Could you check a few things on this model? Use its own coordinates, in mm. A direction names the side the tool comes from. Round coordinates to 2 decimals unless told otherwise and drop trailing zeros. Write each loop counter-clockwise with the first axis right and the second up, starting at its lowest first coordinate (ties: lowest second). Pieces come first, ordered by that corner, then holes. Notation, with made-up numbers: (4.25, -23) - (31.25, -23) arc R28 cw to (31.25, 1) - close; hole circle Ø5 at (-26.75, 16). An arc over 180 degrees is marked (long way). Write each question's results on one line, items separated by ' | '. Start each with the question number.
(1) For P1, Ø2.5, axis at y = 497.5, z = 23.5, coming from the -X side; P2, Ø0.9, axis at y = 539, z = 24.5, coming from the +X side; P3, Ø4, axis at y = 151, z = 21.5, coming from the +X side, each with a flat end and sliding along its axis, tell me the tip position at first contact or that it passes through.
(2) Please list where these lines run through material, in increasing order: line 1 (Z direction, x = 380.5, y = 255); line 2 (X direction, y = 876.5, z = 19); line 3 (X direction, y = 757.5, z = 5.5). Write a range as [from, to].
(3) Imagine slicing it at B-B on y = 354.5. Write out the boundary of the cut face in (x, z), then the cut area to 3 significant figures.
(4) Imagine slicing it at A-A on x = 613. Write out the boundary of the cut face in (y, z).
(5) On a 3-axis mill with a long thin cutter (end or side, diameter ignored), from which of +Z, -Z, +X, -X, +Y, -Y can I reach the whole of each face in a straight line? I mean faces 1 (the flat face through (1002, 618, 25.4)), 2 (the flat face through (664, 618, 3.048)). Say none if no direction works.
(6) Thinking about a two-plate mould opening in Z: for faces 3 (the flat face through (664, 618, 0)), 4 (the flat face through (344, 601, 25.4)), 5 (the flat face through (1011, 618, 22.352)), which applies, +Z half, -Z half, draft (parallel to the pull), parting line (faces both ways), or undercut?
Autodesk Inventor part; units mm, degrees
ref_plane "YZ Plane" through (0, 0, 0) normal (1, 0, 0) x (0, 1, 0)
ref_plane "XZ Plane" through (0, 0, 0) normal (0, 1, 0) x (-1, 0, 0)
ref_plane "XY Plane" through (0, 0, 0) normal (0, 0, 1) x (1, 0, 0)
sketch "Sketch1" plane through (0, 0, 0) normal (0, 0, 1) x (1, 0, 0)
  line L0 (0, 0) -> (1346.2, 0)
  line L1 (1346.2, 0) -> (1346.2, 1219.2)
  line L2 (1346.2, 1219.2) -> (0, 1219.2)
  line L3 (0, 1219.2) -> (0, 0)
  dimension "d0" = 1346.2
  dimension "d1" = 1219.2
extrude "Plate1" add sketch "Sketch1" along normal blind 3.048
sketch "Sketch2" plane through (1343.152, 1219.2, 0) normal (1, 0, 0) x (0, 1, 0)
  line L0 (-1219.2, 0) -> (0, 0)
  line L1 (0, 0) -> (0, 25.4)
  line L2 (0, 25.4) -> (-1219.2, 25.4)
  line L3 (-1219.2, 25.4) -> (-1219.2, 0)
edge flange "Flange1" height 25.4 angle 90 thickness 3.048 bend radius 3.048 thickness toward (1, 0, 0) relief tear relief width 3.048 relief depth 1.524 corner gap 3.048 corner form 0 edges at (1346.2, 609.6, 3.048) (0, 609.6, 3.048) wall of the first edge with corners at (1343.152, 0, 0) (1343.152, 1219.2, 0) (1343.152, 1219.2, 25.4) (1343.152, 0, 25.4)
bend "Bend1"
corner "Corner1"
sketch "Sketch3" plane through (0, 0, 22.352) normal (0, 0, 1) x (1, 0, 0)
  line L0 (0, 1219.2) -> (0, 0)
  line L1 (0, 0) -> (673.099873, 0)
  line L2 (673.099873, 0) -> (673.099873, 1219.2)
  line L3 (673.099873, 1219.2) -> (0, 1219.2)
edge flange "Flange2" height 673.099873 angle 90 thickness 3.048 bend radius 3.048 thickness toward (0, 0, 1) relief tear relief width 3.048 relief depth 1.524 corner gap 3.048 corner form 0 edges at (3.048, 609.6, 25.4) (1343.152, 609.6, 25.4) wall of the first edge with corners at (0, 1219.2, 22.352) (0, 0, 22.352) (673.099873, 0, 22.352) (673.099873, 1219.2, 22.352)
bend "Bend2"
corner "Corner2"
equation "\"d3\" = BendReliefWidth"
equation "\"d4\" = BendReliefDepth"
equation "\"d5\" = MinimumRemnant"
equation "\"d6\" = BendRadius"
equation "\"d9\" = BendRadius"
equation "\"d10\" = CornerReliefSize"
equation "\"d11\" = GapSize"
equation "\"d12\" = JacobiRadiusSize"
equation "\"d13\" = BendReliefWidth"
equation "\"d14\" = BendReliefDepth"
equation "\"d15\" = MinimumRemnant"
equation "\"d16\" = BendRadius"
equation "\"d19\" = BendRadius"
equation "\"d20\" = CornerReliefSize"
equation "\"d21\" = GapSize"
equation "\"d22\" = JacobiRadiusSize"
equation "\"BendRadius\" = Thickness"
equation "\"BendReliefWidth\" = Thickness"
equation "\"BendReliefDepth\" = 0.5 * Thickness"
equation "\"CornerReliefSize\" = 4 * Thickness"
equation "\"MinimumRemnant\" = 2 * Thickness"
equation "\"TransitionRadius\" = BendRadius"
equation "\"JacobiRadiusSize\" = BendRadius"
equation "\"GapSize\" = Thickness"
equation "\"d2\" = BendRadius"
properties part number "top" material "Polycarbonate, Clear"
Response:
1) P1: x = 0.76 | P2: x = 1343.93 | P3: x = 1346.2
2) line 1: [0, 3.05], [22.35, 25.4] | line 2: [0, 3.05], [1343.15, 1346.2] | line 3: [0.03, 3.11], [1343.09, 1346.17]
3) outline: (0, 6.1) arc R6.1 ccw to (6.1, 0) - (1340.1, 0) arc R6.1 ccw to (1346.2, 6.1) - (1346.2, 19.3) arc R6.1 ccw to (1340.1, 25.4) - (673.1, 25.4) - (673.1, 22.35) - (1340.1, 22.35) arc R3.05 cw to (1343.15, 19.3) - (1343.15, 6.1) arc R3.05 cw to (1340.1, 3.05) - (6.1, 3.05) arc R3.05 cw to (3.05, 6.1) - (3.05, 19.3) arc R3.05 cw to (6.1, 22.35) - (673.1, 22.35) - (673.1, 25.4) - (6.1, 25.4) arc R6.1 ccw to (0, 19.3) - close | area: 8,300 mm²
4) outline: (0, 0) - (1219.2, 0) - (1219.2, 3.05) - (0, 3.05) - close; (0, 22.35) - (1219.2, 22.35) - (1219.2, 25.4) - (0, 25.4) - close
5) face 1: +Z, +X, -X, +Y, -Y | face 2: +Y, -Y
6) face 3: -Z half | face 4: +Z half | face 5: undercut
